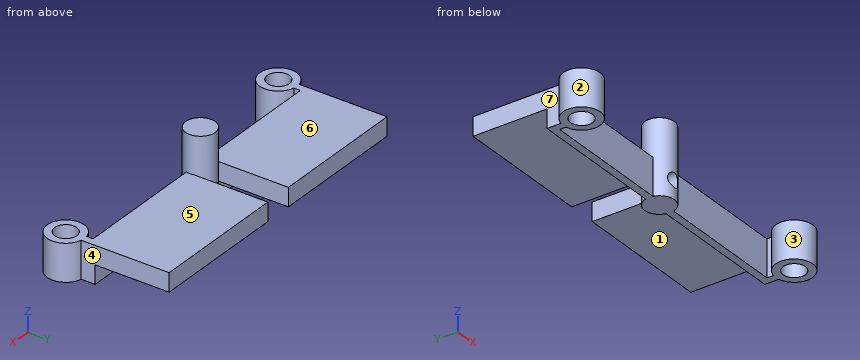
from build123d import *

# Parameters (mm, degrees)
SKETCH1_R                      = 6
BOSS_EXTRUDE1_DEPTH            = 30
SKETCH2_R                      = 4.5
BOSS_EXTRUDE2_DEPTH            = 15
CUT_EXTRUDE1_REACH             = 21
SKETCH3_R                      = 2.868632687
CUT_EXTRUDE1_DIRECTION_2_REACH = 8
SKETCH4_W                      = 55.690524981
SKETCH4_H                      = 7.5
BOSS_EXTRUDE3_DEPTH            = 30


with BuildPart() as part:
    # Sketch1 → Boss-Extrude1 (new body)
    with BuildSketch(Plane.XY):
        Circle(SKETCH1_R)
    extrude(amount=BOSS_EXTRUDE1_DEPTH)

    # Sketch2 → Boss-Extrude2 (add)
    with BuildSketch(Plane.XY):
        with BuildLine():
            Line((6, -1.5), (58.5, -1.5))
            Line((58.5, -1.5), (58.5, -4.151530772))
            ThreePointArc((58.5, -4.151530772), (60, -19), (61.5, -4.151530772))
            Line((61.5, -4.151530772), (61.5, 1.5))
            Line((61.5, 1.5), (6, 1.5))
            Line((6, 1.5), (5.809475019, 1.5))
            ThreePointArc((5.809475019, 1.5), (6, 0), (5.809475019, -1.5))
            Line((5.809475019, -1.5), (6, -1.5))
        make_face()
        with Locations((60, -11.5)):
            Circle(SKETCH2_R, mode=Mode.SUBTRACT)
        with BuildLine():
            Line((-58.5, -1.5), (-58.5, -4.151530772))
            ThreePointArc((-58.5, -4.151530772), (-60, -19), (-61.5, -4.151530772))
            Line((-61.5, -4.151530772), (-61.5, 1.5))
            Line((-61.5, 1.5), (-6, 1.5))
            Line((-6, 1.5), (-5.809475019, 1.5))
            ThreePointArc((-5.809475019, 1.5), (-6, 0), (-5.809475019, -1.5))
            Line((-5.809475019, -1.5), (-6, -1.5))
            Line((-6, -1.5), (-58.5, -1.5))
        make_face()
        with Locations((-60, -11.5)):
            Circle(SKETCH2_R, mode=Mode.SUBTRACT)
    extrude(amount=BOSS_EXTRUDE2_DEPTH)

    # Sketch3 → Cut-Extrude1 (cut, up to next)
    with BuildSketch(Plane(origin=(0, 0, 0), x_dir=(1, 0, 0), z_dir=(0, 1, 0)), mode=Mode.PRIVATE) as cut_extrude1_sk1:
        with Locations((0, -7.5)):
            Circle(SKETCH3_R)
    cut_extrude1_tool1 = extrude(cut_extrude1_sk1.sketch, amount=-CUT_EXTRUDE1_REACH, mode=Mode.PRIVATE) & part.part
    add(cut_extrude1_tool1.solids().sort_by_distance((0, 0, 7.5))[0], mode=Mode.SUBTRACT)

    # Sketch3 → Cut-Extrude1 direction 2 (cut, up to next)
    with BuildSketch(Plane(origin=(0, 0, 0), x_dir=(1, 0, 0), z_dir=(0, 1, 0)), mode=Mode.PRIVATE) as cut_extrude1_direction_2_sk1:
        with Locations((0, -7.5)):
            Circle(SKETCH3_R)
    cut_extrude1_direction_2_tool1 = extrude(cut_extrude1_direction_2_sk1.sketch, amount=CUT_EXTRUDE1_DIRECTION_2_REACH, mode=Mode.PRIVATE) & part.part
    add(cut_extrude1_direction_2_tool1.solids().sort_by_distance((0, 0, 7.5))[0], mode=Mode.SUBTRACT)

    # Sketch4 → Boss-Extrude3 (add)
    with BuildSketch(Plane(origin=(0, 1.5, 0), x_dir=(1, 0, 0), z_dir=(0, 1, 0))):
        with Locations((-33.65473751, -11.25)):
            Rectangle(SKETCH4_W, SKETCH4_H)
        with Locations((33.65473751, -11.25)):
            Rectangle(SKETCH4_W, SKETCH4_H)
    extrude(amount=BOSS_EXTRUDE3_DEPTH)


solid = part.part
Model file for the job. Use its own axes, mm. Face numbers are marked on the shaded views. A direction names the side the tool comes from. Give positions to 0.01 mm unless a question says otherwise; leave off trailing zeros. Loops run counter-clockwise (first coordinate to the right, second up) from the corner with the lowest first, then second, coordinate; pieces in that order, holes last.
1) Saw through at C-C (z = 13). Write the cut outline in (x, y), plus the area to 3 significant figures.
2) Pull direction Y, two halves, no side cores. Call the marked faces 1, 2 and 3: +Y half, -Y half, draft (parallel to the pull), parting line (faces both ways), or undercut.
3) Saw through at B-B (x = 0). Write the cut outline in (y, z).
4) Wall check: line 1 (X direction, y = -11, z = 6); line 2 (X direction, y = -3, z = 7.5); line 3 (X direction, y = -4, z = 14). Give the ranges that are in metal, low to high.
5) Flat gauge pins, fed straight in: pin 1 Ø15 at (x, y) = (44, 18.5) entering from +Z; pin 2 Ø6 at (y, z) = (4, 26) entering from -X; pin 3 Ø4 at (y, z) = (9, 14.5) entering from -X. Where does each tip first touch, or does it go through?
6) Saw through at A-A (y = 0). Write the cut outline in (x, z), plus the area to 3 significant figures.
7) Saw through at D-D (y = 24.5). Write the cut outline in (x, z).
8) Tool access for the marked faces 4, 5, 6 and 7: list every direction of +Z, -Z, +X, -X, +Y, -Y with a clear straight run to the whole face (end or side of a thin tool).
Answer block:
1. outline: (-61.5, -4.15) arc R7.5 ccw (long way) to (-58.5, -4.15) - (-58.5, -1.5) - (-5.81, -1.5) arc R6 ccw to (5.81, -1.5) - (58.5, -1.5) - (58.5, -4.15) arc R7.5 ccw (long way) to (61.5, -4.15) - (61.5, 31.5) - (5.81, 31.5) - (5.81, 1.5) arc R6 ccw to (-5.81, 1.5) - (-5.81, 31.5) - (-61.5, 31.5) - close; hole circle Ø9 at (-60, -11.5); hole circle Ø9 at (60, -11.5)
1. area: 4,030 mm2
2. face 1: draft
2. face 2: undercut
2. face 3: undercut
3. outline: (-6, 0) - (6, 0) - (6, 4.63) - (-6, 4.63) - close; (-6, 10.37) - (6, 10.37) - (6, 30) - (-6, 30) - close
4. line 1: x = -67.48 to -64.47, -55.53 to -52.52, 52.52 to 55.53, 64.47 to 67.48
4. line 2: x = -61.5 to -58.5, -5.2 to -2.87, 2.87 to 5.2, 58.5 to 61.5
4. line 3: x = -61.5 to -58.5, -4.47 to 4.47, 58.5 to 61.5
5. pin 1: stops at z = 15
5. pin 2: stops at x = -5.92
5. pin 3: stops at x = -61.5
6. outline: (-61.5, 0) - (61.5, 0) - (61.5, 15) - (6, 15) - (6, 30) - (-6, 30) - (-6, 15) - (-61.5, 15) - close; hole circle Ø5.74 at (0, 7.5)
6. area: 2,000 mm2
7. outline: (-61.5, 7.5) - (-5.81, 7.5) - (-5.81, 15) - (-61.5, 15) - close; (5.81, 7.5) - (61.5, 7.5) - (61.5, 15) - (5.81, 15) - close
8. face 4: +Z, -Z, +X, +Y
8. face 5: +Z, +X, +Y, -Y
8. face 6: +Z, -X, +Y, -Y
8. face 7: +Z, -Z, -X, +Y
